The model under review builds one solid part; all positions refer to its coordinate system, in mm. A direction names the side the tool comes from. Round coordinates to 2 decimals unless told otherwise and drop trailing zeros. Order: outer loops, then holes, each group sorted by start corner. A loop starts at its lowest first (then second) coordinate and runs counter-clockwise, first axis right, second up.
```python
from build123d import *

# Parameters (mm, degrees)
ESQUISSE1_W               = 47
ESQUISSE1_H               = 23
BOSS_EXTRU_1_DEPTH        = 10
TROU_TARAUD_M1_4X0_32_D   = 1.1
ESQUISSE5_W               = 20
ESQUISSE5_H               = 15
ENL_V_MAT_EXTRU_1_DEPTH   = 10
ESQUISSE6_W               = 20
ESQUISSE6_H               = 10.927419914
BOSS_EXTRU_2_DEPTH        = 20
ESQUISSE9_W               = 20
ESQUISSE9_H               = 10
BOSS_EXTRU_5_DEPTH        = 20
ESQUISSE10_R              = 10
BOSS_EXTRU_6_DEPTH        = 20
TROU_TARAUD_M5X0_81_D     = 4.2
TROU_TARAUD_M5X0_81_DEPTH = 10
TROU_TARAUD_M5X0_81_TIP   = 1.2618073


with BuildPart() as part:
    # Esquisse1 → Boss.-Extru.1 (new body)
    with BuildSketch(Plane.XY):
        Rectangle(ESQUISSE1_W, ESQUISSE1_H)
    extrude(amount=BOSS_EXTRU_1_DEPTH)

    # Trou taraudé M1.4x0.32 (through all)
    with Locations(Plane(origin=(-21, 8.5, 10), x_dir=(1, 0, 0), z_dir=(0, 0, 1))):
        with Locations((0, 0), (0, -17), (42, -17), (42, 0)):
            Hole(TROU_TARAUD_M1_4X0_32_D / 2)

    # Esquisse5 → Enlèv. mat.-Extru.1 (cut)
    with BuildSketch(Plane.XY.offset(10)):
        with Locations((0, -6.927419914)):
            Rectangle(ESQUISSE5_W, ESQUISSE5_H)
    extrude(amount=-ENL_V_MAT_EXTRU_1_DEPTH, mode=Mode.SUBTRACT)

    # Esquisse6 → Boss.-Extru.2 (add)
    with BuildSketch(Plane(origin=(0, 0, 0), x_dir=(-1, 0, 0), z_dir=(0, 0, -1))):
        with Locations((0, 6.036290043)):
            Rectangle(ESQUISSE6_W, ESQUISSE6_H)
    extrude(amount=BOSS_EXTRU_2_DEPTH)

    # Esquisse9 → Boss.-Extru.5 (add)
    with BuildSketch(Plane(origin=(0, 11.5, 0), x_dir=(1, 0, 0), z_dir=(0, 1, 0))):
        with Locations((0, 15)):
            Rectangle(ESQUISSE9_W, ESQUISSE9_H)
    extrude(amount=BOSS_EXTRU_5_DEPTH)

    # Esquisse10 → Boss.-Extru.6 (add)
    with BuildSketch(Plane(origin=(0, 31.5, 0), x_dir=(1, 0, 0), z_dir=(0, 1, 0))):
        with Locations(Location((0, 15, 0), (0, 0, 30))):
            Circle(ESQUISSE10_R)
    extrude(amount=BOSS_EXTRU_6_DEPTH)

    # Trou taraudé M5x0.81
    with Locations(Plane(origin=(0, 51.5, -15), x_dir=(0, 0, 1), z_dir=(0, 1, 0))):
        with Locations((0, 0)):
            Hole(TROU_TARAUD_M5X0_81_D / 2, depth=TROU_TARAUD_M5X0_81_DEPTH)
            with Locations((0, 0, -(TROU_TARAUD_M5X0_81_DEPTH + TROU_TARAUD_M5X0_81_TIP / 2))):  # 118° drill point
                Cone(0, TROU_TARAUD_M5X0_81_D / 2, TROU_TARAUD_M5X0_81_TIP, mode=Mode.SUBTRACT)


solid = part.part
```
(1) Consider section C-C (z = -23). Write out the cut boundary in (x, y), and give its area (3 significant figures).
Data:
outline: (-6, 31.5) - (6, 31.5) - (6, 51.5) - (-6, 51.5) - close
area: 240 mm2
(2) For faces 1 (the flat face through (0, 31.5, -22)), 2 (the flat face through (0, 21, -10)), 3 (the flat face through (9.5, 31.5, -11.2)), list the 3-axis set-ups (+Z, -Z, +X, -X, +Y, -Y) from which the entire face can be reached by the end or side of a thin tool; tool diameter is ignored.
Data:
face 1: -Z, +X, -X, -Y
face 2: +Z, +X, -X
face 3: +Z, +X, +Y
(3) Insertion check: pin 1 (5 mm diameter, centred on x = 5.5, y = 40.5, fed in from +Z); pin 2 (3 mm diameter, centred on x = -13, y = 6, fed in from -Z); pin 3 (16 mm diameter, centred on x = 0, y = 24.5, fed in from +Z). Each pin has a flat end and moves straight along its axis. Give the tip position at first contact, or say it passes through.
Data:
pin 1: stops at z = -5.46
pin 2: stops at z = 0
pin 3: stops at z = -5
(4) Consider section B-B (x = 14). Write out the cut boundary in (y, z), and give its area (3 significant figures).
Data:
outline: (-11.5, 0) - (11.5, 0) - (11.5, 10) - (-11.5, 10) - close
area: 230 mm2
(5) To check wall thickness, follow probe 1 along Y at (x, z) = (21, 3); probe 2 along Z at (x, y) = (0, 44); probe 3 along Z at (x, y) = (-16, -9). State the ranges of each line that lie inside material, in increasing order.
Data:
probe 1: y = -11.5 to -9.05, -7.95 to 7.95, 9.05 to 11.5
probe 2: z = -25 to -17.1, -12.9 to -5
probe 3: z = 0 to 10
(6) Consider section D-D (y = 39). Write out the cut boundary in (x, z), and give its area (3 significant figures).
Data:
outline: circle Ø20 at (0, -15)
area: 314 mm2
(7) Consider section A-A (y = 6.5). Write out the cut boundary in (x, z), and give its area (3 significant figures).
Data:
outline: (-23.5, 0) - (-10, 0) - (-10, -20) - (10, -20) - (10, 0) - (23.5, 0) - (23.5, 10) - (-23.5, 10) - close
area: 870 mm2
(8) Draft analysis for pull direction Z (two halves, no side actions). For faces 4 (the cylindrical face through (0.09, 46.43, -12.9)), 5 (the cylindrical face through (-3.83, 41.36, -5.763)), 6 (the flat face through (10, -6, 5)), state which applies: pulls with the +Z half, pulls with the -Z half, needs draft (parallel to the pull), parting line crosses it, or undercut.
Data:
face 4: undercut
face 5: parting line crosses it
face 6: needs draft
